```python
from build123d import *

# Parameters (mm, degrees)
F1_DEPTH = 1.5
F2_DEPTH = 4.5


# Not quite as in the source:
# - a feature names something its author has since deleted; it is built from what else it names


with BuildPart() as f1:
    # F0 (on Top) → F1 (new body)
    with BuildSketch(Plane.XY):
        with BuildLine():
            ThreePointArc((2.25, -3), (3.3541019662, -1.6770509831), (3.75, 0))
            ThreePointArc((3.75, 0), (3.3541019662, 1.6770509831), (2.25, 3))
            ThreePointArc((2.25, 3), (-3.75, 0), (2.25, -3))
        make_face()
        with BuildLine():
            ThreePointArc((16.75, 0), (16.2191802202, 1.3570222845), (14.9084905194, 1.9937102987))
            ThreePointArc((14.9084905194, 1.9937102987), (12.75, 0), (14.9084905194, -1.9937102987))
            ThreePointArc((14.9084905194, -1.9937102987), (16.2191802202, -1.3570222845), (16.75, 0))
        make_face()
        with BuildLine():
            ThreePointArc((2.25, 3), (3.3541019662, 1.6770509831), (3.75, 0))
            ThreePointArc((3.75, 0), (3.3541019662, -1.6770509831), (2.25, -3))
            Line((2.25, -3), (14.9084905194, -1.9937102987))
            ThreePointArc((14.9084905194, -1.9937102987), (12.75, 0), (14.9084905194, 1.9937102987))
            Line((14.9084905194, 1.9937102987), (2.25, 3))
        make_face()
    extrude(amount=F1_DEPTH)

    # F0 (on Top) → F2 (join)
    with BuildSketch(Plane.XY):
        with BuildLine():
            ThreePointArc((2.25, -3), (3.3541019662, -1.6770509831), (3.75, 0))
            ThreePointArc((3.75, 0), (3.3541019662, 1.6770509831), (2.25, 3))
            ThreePointArc((2.25, 3), (-3.75, 0), (2.25, -3))
        make_face()
    extrude(amount=F2_DEPTH)


solid = f1.part
```
Verification items for the finished model (mm, model axes). Coordinates: 2 decimals unless noted, no trailing zeros. Order: outer loops, then holes, each group sorted by start corner. A loop starts at its lowest first (then second) coordinate and runs counter-clockwise, first axis right, second up. Notation, with made-up numbers: (75.25, -19.5) -> (127.25, -19.5) arc R7 ccw to (127.25, -10.5) -> close; hole circle Ø2 at (18.5, -7). An arc over 180 degrees is marked (long way). Put each result on its own line as item: value. Start each with the question number.
1) Release check for a two-part mould opening along X. For faces 1 (the flat face through (6, 0, 0)), 2 (the flat face through (8.491, -2.504, 0.74)), 3 (the cylindrical face through (-3.61, 1.01, 2.22)) record: pulls with the +X half, pulls with the -X half, needs draft (parallel to the pull), parting line crosses it, or undercut.
2) Go/stop test with flat-tipped pins: pin 1 (1.5 mm diameter, centred on x = 6, y = 2, fed in from +Z); pin 2 (1.5 mm diameter, centred on y = 2, z = 4, fed in from +X); pin 3 (2 mm diameter, centred on x = 6.5, z = 3, fed in from +Y); pin 4 (2 mm diameter, centred on y = 2, z = 0.5, fed in from -X). Record where each tip stops, or that it passes through.
3) Cross-section at A-A (z = 4.05). Enter the section's corners in (x, y), plus the area to 3 significant figures.
4) Cross-section at D-D (y = 2.5). Enter the section's corners in (x, z), plus the area to 3 significant figures.
5) Cross-section at B-B (y = 0.5). Enter the section's corners in (x, z).
6) Cross-section at C-C (x = 13.75). Enter the section's corners in (y, z).
7) Material ranges on L1, parallel to Z at x = 7.25, y = 0.25; L2, parallel to Y at x = 10.25, z = 0.6; L3, parallel to X at y = 1, z = 2.9, recorded low to high.
Geometry check:
1. face 1: needs draft
1. face 2: pulls with the +X half
1. face 3: parting line crosses it
2. pin 1: stops at z = 1.5
2. pin 2: stops at x = 3.54
2. pin 3: passes through
2. pin 4: stops at x = -3.61
3. outline: circle Ø7.5 at (0, 0)
3. area: 44.2 mm^2
4. outline: (-2.8, 0) -> (8.54, 0) -> (8.54, 1.5) -> (2.8, 1.5) -> (2.8, 4.5) -> (-2.8, 4.5) -> close
4. area: 33.8 mm^2
5. outline: (-3.72, 0) -> (16.69, 0) -> (16.69, 1.5) -> (3.72, 1.5) -> (3.72, 4.5) -> (-3.72, 4.5) -> close
6. outline: (-2.09, 0) -> (2.09, 0) -> (2.09, 1.5) -> (-2.09, 1.5) -> close
7. L1: z = 0 to 1.5
7. L2: y = -2.36 to 2.36
7. L3: x = -3.61 to 3.61
